Source: three-view drawing plus pictorial views. Frame: mm from the lowest corner of the part. A direction names the side the tool comes from. Give positions to 0.01 mm unless a question says otherwise; leave off trailing zeros. Loops run counter-clockwise (first coordinate to the right, second up) from the corner with the lowest first, then second, coordinate; pieces in that order, holes last. Notation, with made-up numbers: (16, 71.25) -> (74, 71.25) arc R20 cw to (74, 102.25) -> close; hole circle Ø5 at (-36.75, 18). An arc over 180 degrees is marked (long way). Put each result on its own line as item: value.
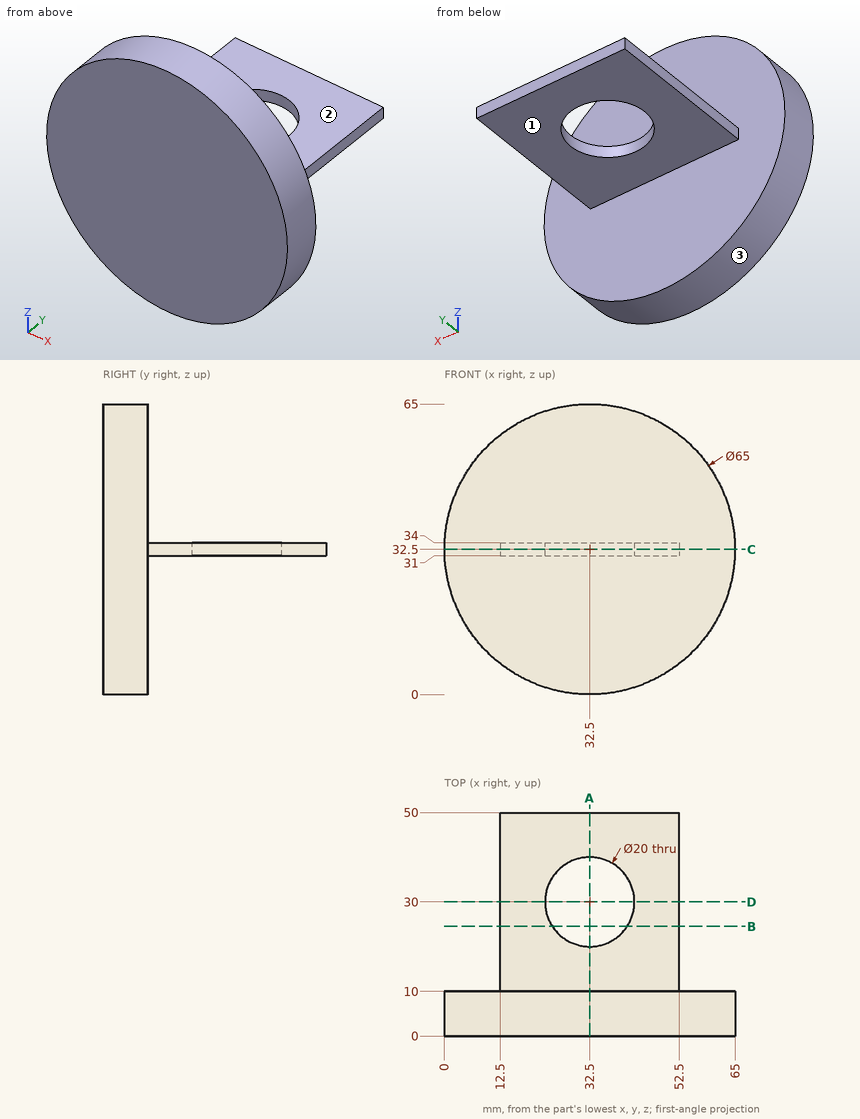
(1) Reachability of the marked faces 1, 2 and 3 from +Z, -Z, +X, -X, +Y, -Y: full face, straight path, thin tool, end or side. Return the list, or none.
Calculated:
face 1: -Z, +X, -X, +Y
face 2: +Z, +X, -X, +Y
face 3: +Y, -Y
(2) Section C-C on z = 32.5. Return loops of the section in (x, y), then the cut area to 3 significant figures.
Calculated:
outline: (0, 0) -> (65, 0) -> (65, 10) -> (52.5, 10) -> (52.5, 50) -> (12.5, 50) -> (12.5, 10) -> (0, 10) -> close; hole circle Ø20 at (32.5, 30)
area: 1,940 mm²
(3) Line query: probe 1 along Y at (x, z) = (32.5, 31.9); probe 2 along Z at (x, y) = (14.5, 25); probe 3 along Y at (x, z) = (49.5, 49). Output: solid intervals per line, ascending. Write a range as from..to.
Calculated:
probe 1: y = 0..20, 40..50
probe 2: z = 31..34
probe 3: y = 0..10
(4) Section A-A on x = 32.5. Return loops of the section in (y, z).
Calculated:
outline: (0, 0) -> (10, 0) -> (10, 31) -> (20, 31) -> (20, 34) -> (10, 34) -> (10, 65) -> (0, 65) -> close; (40, 31) -> (50, 31) -> (50, 34) -> (40, 34) -> close
(5) First-contact query: P1, Ø5, axis at x = 9, y = 21.5, coming from the +Z side; P2, Ø2.5, axis at y = 40, z = 32, coming from the -X side; P3, Ø3.5, axis at y = 33, z = 32.5, coming from the +X side; P4, Ø8, axis at x = 26.5, y = 40, coming from the +Z side. Flat tips, straight axial feed; report the tip coordinate or a pass-through.
Calculated:
P1: passes through
P2: stops at x = 12.5
P3: stops at x = 52.5
P4: stops at z = 34
(6) Section D-D on y = 30. Return loops of the section in (x, z).
Calculated:
outline: (12.5, 31) -> (22.5, 31) -> (22.5, 34) -> (12.5, 34) -> close; (42.5, 31) -> (52.5, 31) -> (52.5, 34) -> (42.5, 34) -> close
(7) Section B-B on y = 24.5. Return loops of the section in (x, z).
Calculated:
outline: (12.5, 31) -> (24.15, 31) -> (24.15, 34) -> (12.5, 34) -> close; (40.85, 31) -> (52.5, 31) -> (52.5, 34) -> (40.85, 34) -> close
